Solid Edge part; units mm, degrees
sketch "Sketch1" plane through (0, 0, 0) normal (0, 0, 1) x (1, 0, 0)
  circle A0 centre (0, 0) radius 3.15
extrude "Protrusion1" add sketch "Sketch1" against normal blind 9
sketch "Sketch2" plane through (0, 0, -9) normal (0, 0, -1) x (1, 0, 0)
  circle A0 centre (0, 0) radius 3.15
extrude "ExtrudedProtrusion_2" add sketch "Sketch2" along normal blind 10.4
sketch "Sketch3" plane through (0, 0, -19.4) normal (0, 0, -1) x (1, 0, 0)
  circle A0 centre (0, 0) radius 19.05
extrude "ExtrudedProtrusion_3" add sketch "Sketch3" along normal blind 1.7
sketch "Sketch4" plane through (0, 0, -21.1) normal (0, 0, -1) x (1, 0, 0)
  circle A0 centre (23.55, 23.55) radius 2.5
  circle A1 centre (23.55, -23.55) radius 2.5
  circle A2 centre (-23.55, -23.55) radius 2.5
  circle A3 centre (-23.55, 23.55) radius 2.5
  line L0 (-25.4, -28.2) -> (25.4, -28.2)
  arc A4 (28.2, -25.4) -> (25.4, -28.2) centre (25.4, -25.4) cw
  line L1 (28.2, -25.4) -> (28.2, 25.4)
  arc A5 (25.4, 28.2) -> (28.2, 25.4) centre (25.4, 25.4) cw
  line L2 (25.4, 28.2) -> (-25.4, 28.2)
  arc A6 (-28.2, 25.4) -> (-25.4, 28.2) centre (-25.4, 25.4) cw
  line L3 (-28.2, 25.4) -> (-28.2, -25.4)
  arc A7 (-25.4, -28.2) -> (-28.2, -25.4) centre (-25.4, -25.4) cw
extrude "ExtrudedProtrusion_4" add sketch "Sketch4" along normal blind 5.2
sketch "Sketch5" plane through (0, 0, -26.3) normal (0, 0, -1) x (0, -1, 0)
  line L0 (-28.2, 19.8235) -> (-28.2, -19.8235)
  line L1 (-19.8235, -28.2) -> (19.8235, -28.2)
  line L2 (28.2, -19.8235) -> (28.2, 19.8235)
  line L3 (19.8235, 28.2) -> (-19.8235, 28.2)
  arc A0 (-28.2, -19.8235) -> (-19.8235, -28.2) centre (-23.3345, -23.3345) cw
  arc A1 (19.8235, -28.2) -> (28.2, -19.8235) centre (23.3345, -23.3345) cw
  arc A2 (28.2, 19.8235) -> (19.8235, 28.2) centre (23.3345, 23.3345) cw
  arc A3 (-19.8235, 28.2) -> (-28.2, 19.8235) centre (-23.3345, 23.3345) cw
extrude "ExtrudedProtrusion_5" add sketch "Sketch5" along normal blind 46.1
sketch "Sketch6" plane through (0, 0, -72.4) normal (0, 0, -1) x (-1, 0, 0)
  circle A0 centre (0, 0) radius 3.15
extrude "ExtrudedProtrusion_6" add sketch "Sketch6" along normal blind 13.3
sketch "Sketch7" plane through (0, 0, 0) normal (0, -1, 0) x (1, 0, 0)
  line L0 (0, -5.9) -> (23.1327, -5.9)
extrude "Cutout1" cut sketch "Sketch7" along normal through all and the other way through all material side at (11.5663, 0, -5.85)
properties material "Stainless steel"
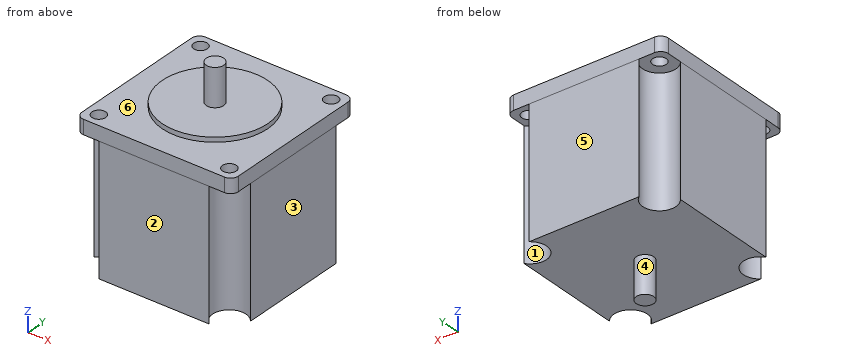
Could you check a few things on this model? Use its own coordinates, in mm. Face numbers are marked on the shaded views. A direction names the side the tool comes from. Round coordinates to 2 decimals unless told otherwise and drop trailing zeros. Loops run counter-clockwise (first coordinate to the right, second up) from the corner with the lowest first, then second, coordinate; pieces in that order, holes last. Notation, with made-up numbers: (-9, -9) - (34, -9) arc R18 cw to (34, 19) - close; hole circle Ø2 at (10, 78). An arc over 180 degrees is marked (long way). Use CSV: the item, a comma, the result in double quotes.
Item 1: Will these pins go through, and if not, where does the flat tip stop? pin 1 (4 mm diameter, centred on x = -6, y = -9.5, fed in from +Z); pin 2 (6.5 mm diameter, centred on x = -23.55, y = 23.55, fed in from -Z); pin 3 (12 mm diameter, centred on x = -1, z = -76, fed in from +Y); pin 4 (19 mm diameter, centred on x = -23.33, y = -23.33, fed in from -Z).
Here are the results:
pin 1,"stops at z = -19.4"
pin 2,"stops at z = -26.3"
pin 3,"stops at y = 28.2"
pin 4,"stops at z = -72.4"
Item 2: If we section it at A-A on x = 23.55: List the corners of the cut face in (y, z) for me, then the cut area to 3 significant figures.
Here are the results:
outline,"(-28.2, -26.3) - (-26.05, -26.3) - (-26.05, -21.1) - (-28.2, -21.1) - close; (-21.05, -26.3) - (-17.34, -26.3) - (-17.34, -72.4) - (17.34, -72.4) - (17.34, -26.3) - (21.05, -26.3) - (21.05, -21.1) - (-21.05, -21.1) - close; (26.05, -26.3) - (28.2, -26.3) - (28.2, -21.1) - (26.05, -21.1) - close"
area,"1,840 mm²"
Item 3: If we section it at B-B on z = -24.5: List the corners of the cut face in (x, y) for me.
Here are the results:
outline,"(-28.2, -25.4) arc R2.8 ccw to (-25.4, -28.2) - (25.4, -28.2) arc R2.8 ccw to (28.2, -25.4) - (28.2, 25.4) arc R2.8 ccw to (25.4, 28.2) - (-25.4, 28.2) arc R2.8 ccw to (-28.2, 25.4) - close; hole circle Ø5 at (-23.55, -23.55); hole circle Ø5 at (-23.55, 23.55); hole circle Ø5 at (23.55, -23.55); hole circle Ø5 at (23.55, 23.55)"
Item 4: If we mould it in two halves opening along X, with no side actions, what happens to the marked faces 1, 2 and 3? For each: pulls with the +X half, pulls with the -X half, needs draft (parallel to the pull), parting line crosses it, or undercut.
Here are the results:
face 1,"undercut"
face 2,"needs draft"
face 3,"pulls with the +X half"
Item 5: I need wall thicknesses on L1, parallel to X at y = -19.5, z = -52; L2, parallel to Y at x = -23.55, z = -22.9; L3, parallel to Z at x = 25.5, y = 5. Which ranges of each line are inside material? Lowest first, please. Write a range as [from, to].
Here are the results:
L1,"x = [-28.2, -27.95], [-18.72, 18.72], [27.95, 28.2]"
L2,"y = [-28.2, -26.05], [-21.05, 21.05], [26.05, 28.2]"
L3,"z = [-72.4, -21.1]"
Item 6: For the marked faces 4, 5 and 6, which set-ups out of +Z, -Z, +X, -X, +Y, -Y let a thin tool reach every point of the face, with its end or its side?
Here are the results:
face 4,"-Z"
face 5,"+Z, -Z, +X, -X, +Y"
face 6,"+Z"
